The model under review builds one solid part; all positions refer to its coordinate system, in mm. A direction names the side the tool comes from. Round coordinates to 2 decimals unless told otherwise and drop trailing zeros. Return JSON: item names as keys, results as strings. Group by question number.
```python
from build123d import *

# Parameters (mm, degrees)
SKETCH1_R               = 4.7625
BOSS_EXTRUDE2_DEPTH     = 30.48
FILLET1_R               = 3.175
FILLET3_R               = 1.27
FILLET4_R               = 3.175
FILLET5_R               = 1.27
FILLET6_R               = 1.27
BOSS_EXTRUDE9_START     = -30.48
BOSS_EXTRUDE9_DEPTH     = 30.48
CUT_EXTRUDE6_START      = -30.48
CUT_EXTRUDE6_DEPTH      = 30.48
FILLET9_R               = 6.35
CUT_EXTRUDE7_DEPTH      = 44.536935081
CUT_EXTRUDE7_DEPTH_BACK = 44.536935081
BOSS_EXTRUDE11_START    = -30.48
SKETCH4_R               = 4.7625
BOSS_EXTRUDE11_DEPTH    = 30.48
FILLET10_R              = 12.7
FILLET11_R              = 12.7


with BuildPart() as part:
    # Sketch1 → Boss-Extrude2 (new body)
    with BuildSketch(Plane(origin=(0, 0, 0), x_dir=(1, 0, 0), z_dir=(0, 1, 0))):
        with BuildLine():
            Line((11.860213807, -12.884548704), (13.754545104, -18.945407466))
            Line((13.754545104, -18.945407466), (7.404545104, -18.945407466))
            Line((7.404545104, -18.945407466), (6.640447212, -16.500698134))
            ThreePointArc((6.640447212, -16.500698134), (5.961240353, -16.792309403), (5.2705, -17.055438375))
            ThreePointArc((5.2705, -17.055438375), (0, -22.325938375), (-5.2705, -17.055438375))
            ThreePointArc((-5.2705, -17.055438375), (-5.919586773, -14.929400926), (-6.188032569, -12.722755117))
            ThreePointArc((-6.188032569, -12.722755117), (-14.1478, 0), (-6.188032569, 12.722755117))
            ThreePointArc((-6.188032569, 12.722755117), (-5.919586773, 14.929400926), (-5.2705, 17.055438375))
            ThreePointArc((-5.2705, 17.055438375), (0, 22.325938375), (5.2705, 17.055438375))
            ThreePointArc((5.2705, 17.055438375), (12.040379738, 12.314885712), (16.362502035, 5.2705))
            ThreePointArc((16.362502035, 5.2705), (21.633002035, 0), (16.362502035, -5.2705))
            ThreePointArc((16.362502035, -5.2705), (14.592418813, -9.361982053), (11.860213807, -12.884548704))
        make_face()
        with Locations(Location((0, 17.055438375, 0), (0, 0, 90))):
            Circle(SKETCH1_R, mode=Mode.SUBTRACT)
        with Locations(Location((16.362502035, 0, 0), (0, 0, 90))):
            Circle(SKETCH1_R, mode=Mode.SUBTRACT)
        with Locations(Location((0, -17.055438375, 0), (0, 0, 90))):
            Circle(SKETCH1_R, mode=Mode.SUBTRACT)
        with BuildLine():
            Line((5.737156066, -9.353468881), (8.338191551, -17.675407466))
            Line((8.338191551, -17.675407466), (12.027017511, -17.675407466))
            Line((12.027017511, -17.675407466), (8.623309815, -6.785342119))
            ThreePointArc((8.623309815, -6.785342119), (-7.294145861, 8.197424961), (5.737156066, -9.353468881))
        make_face(mode=Mode.SUBTRACT)
    extrude(amount=BOSS_EXTRUDE2_DEPTH)

    # Fillet1
    # the kernel refuses this fillet: 3.175 mm, written as the material it adds along each edge
    with BuildSketch(Plane(origin=(-6.188032569, 0, -12.722755117), x_dir=(-0.8747186698844794, 0, 0.4846310437389738), z_dir=(0, 1, 0))) as fillet1_piece_1:
        with BuildLine():
            CenterArc((1.675106808, -3.170499128), FILLET1_R, 93.05116293, 49.316383357)
            ThreePointArc((-0.839315123, -1.231863693), (-0.401568779, -0.628256415), (0, 0))
            ThreePointArc((0, 0), (0.753054473, -0.020055884), (1.506108946, 0))
        make_face()
    extrude(amount=30.48)
    with BuildSketch(Plane(origin=(-5.2705, 0, -17.055438375), x_dir=(-0.35770128840140486, 0, 0.9338360607065755), z_dir=(0, 1, 0))) as fillet1_piece_2:
        with BuildLine():
            CenterArc((0.51828136, -3.174477714), FILLET1_R, 91.039263795, 15.495369937)
            ThreePointArc((-0.385307362, -0.130770695), (-0.191391238, -0.069105054), (0, 0))
            ThreePointArc((0, 0), (0.230347271, -0.002089143), (0.460694542, 0))
        make_face()
    extrude(amount=30.48)
    with BuildSketch(Plane(origin=(5.2705, 0, -17.055438375), x_dir=(-0.12720688847868244, 0, -0.9918762057452392), z_dir=(0, 1, 0))) as fillet1_piece_3:
        with BuildLine():
            CenterArc((1.744769682, -3.149206953), FILLET1_R, 97.308218729, 47.663807195)
            ThreePointArc((-0.855148612, -1.326832167), (-0.414685297, -0.671723102), (0, 0))
            ThreePointArc((0, 0), (0.670443906, -0.042816458), (1.340887811, 0))
        make_face()
    extrude(amount=30.48)
    with BuildSketch(Plane(origin=(16.362502035, 0, -5.2705), x_dir=(-0.3771647323765371, 0, -0.9261461896759794), z_dir=(0, 1, 0))) as fillet1_piece_4:
        with BuildLine():
            CenterArc((1.804499427, -3.172306197), FILLET1_R, 92.360366346, 49.97819677)
            ThreePointArc((-0.70894152, -1.232399084), (-0.312723775, -0.640214629), (0, 0))
            ThreePointArc((0, 0), (0.8368693, -0.017240341), (1.673738599, 0))
        make_face()
    extrude(amount=30.48)
    with BuildSketch(Plane(origin=(16.362502035, 0, 5.2705), x_dir=(0.9898341628287173, 0, -0.14222633404954374), z_dir=(0, 1, 0))) as fillet1_piece_5:
        with BuildLine():
            CenterArc((1.950776398, -3.142723467), FILLET1_R, 98.176695151, 51.81827723)
            ThreePointArc((-0.798714948, -1.554982197), (-0.380235314, -0.787313176), (0, 0))
            ThreePointArc((0, 0), (0.749603894, -0.053579045), (1.499207787, 0))
        make_face()
    extrude(amount=30.48)
    with BuildSketch(Plane(origin=(11.860213807, 0, 12.884548704), x_dir=(0.29831988928740816, 0, 0.9544659468286695), z_dir=(0, 1, 0))) as fillet1_piece_6:
        with BuildLine():
            CenterArc((1.816465361, 3.175), FILLET1_R, 213.037149694, 56.962850306)
            ThreePointArc((-0.845191928, 1.444044923), (-0.405599886, 0.731970177), (0, 0))
            Line((0, 0), (1.816465361, 0))
        make_face()
    extrude(amount=30.48)
    with BuildSketch(Plane(origin=(5.2705, 0, 17.055438375), x_dir=(0.9268908474954334, 0, -0.37533099636080863), z_dir=(0, 1, 0))) as fillet1_piece_7:
        with BuildLine():
            CenterArc((1.820147869, -3.156511003), FILLET1_R, 96.186334825, 46.370096176)
            ThreePointArc((-0.700651409, -1.226175281), (-0.30907029, -0.636661485), (0, 0))
            ThreePointArc((0, 0), (0.73900137, -0.015364429), (1.47800274, 0))
        make_face()
    extrude(amount=30.48)
    with BuildSketch(Plane(origin=(-5.2705, 0, 17.055438375), x_dir=(0.038601082712793416, 0, 0.999254700471006), z_dir=(0, 1, 0))) as fillet1_piece_8:
        with BuildLine():
            CenterArc((0.52945245, -3.172633674), FILLET1_R, 92.212228742, 15.495369937)
            ThreePointArc((-0.436253651, -0.148061518), (-0.217455401, -0.076009068), (0, 0))
            ThreePointArc((0, 0), (0.203447006, -0.003928101), (0.406894013, 0))
        make_face()
    extrude(amount=30.48)
    # the kernel refuses this fillet: 3.175 mm, written as the material it takes off along each edge
    with BuildSketch(Plane(origin=(5.737156066, -8.75064331, 9.353468881), x_dir=(0.29831988928740744, 0, 0.9544659468286697), z_dir=(0, 1, 0))) as fillet1_2_piece_1:
        with BuildLine():
            CenterArc((3.500257324, -3.175), FILLET1_R, 90, 88.017608619)
            ThreePointArc((0.327157544, -3.065169276), (0.271751922, -1.521038893), (0, 0))
            Line((0, 0), (3.500257324, 0))
        make_face()
    extrude(amount=47.98128662, mode=Mode.SUBTRACT)

    # Fillet3
    fillet3_edges = [part.edges().sort_by_distance(p)[0] for p in [
        (13.754545104, 15.24, 18.945407466),
        (7.404545104, 15.24, 18.945407466),
    ]]
    fillet(fillet3_edges, radius=FILLET3_R)

    # Fillet4
    # the kernel refuses this fillet: 3.175 mm, written as the material it adds along each edge
    with BuildSketch(Plane(origin=(12.027017511, 0, 17.675407466), x_dir=(-0.29831988928740777, 0, -0.9544659468286695), z_dir=(0, 1, 0))) as fillet4_piece_1:
        with BuildLine():
            CenterArc((4.256556411, 3.175), FILLET4_R, 173.746252409, 96.253747591)
            Line((1.100450152, 3.520858762), (1.037328027, 3.527775938))
            ThreePointArc((1.037328027, 3.527775938), (0.489616488, 1.779372694), (-0.060608588, 0.018943313))
            Line((-0.060608588, 0.018943313), (0, -0.0635))
            Line((0, -0.0635), (4.256556411, -0.0635))
            Line((4.256556411, -0.0635), (4.256556411, 0))
        make_face()
    extrude(amount=30.48)

    # Fillet5
    fillet5_edges = [part.edges().sort_by_distance(p)[0] for p in [
        (8.338191551, 15.24, 17.675407466),
    ]]
    fillet(fillet5_edges, radius=FILLET5_R)

    # Fillet6
    fillet6_edges = [part.edges().sort_by_distance(p)[0] for p in [
        (6.640447212, 15.24, 16.500698134),
        (8.623309815, 15.24, 6.785342119),
    ]]
    fillet(fillet6_edges, radius=FILLET6_R)

    # Sketch2 → Boss-Extrude9 (add)
    with BuildSketch(Plane(origin=(0, 30.48, 0), x_dir=(1, 0, 0), z_dir=(0, 1, 0)).offset(BOSS_EXTRUDE9_START)):
        with BuildLine():
            ThreePointArc((7.943426233, 15.662766674), (13.175324303, 14.973004025), (15.611766116, 10.291948459))
            ThreePointArc((15.611766116, 10.291948459), (15.492196473, 9.129027942), (15.138490831, 8.014768839))
            ThreePointArc((15.138490831, 8.014768839), (15.444654673, 7.422560084), (15.731226864, 6.820626626))
            ThreePointArc((15.731226864, 6.820626626), (15.781158654, 6.716236617), (15.834861283, 6.61373547))
            ThreePointArc((15.834861283, 6.61373547), (16.614943687, 8.379799111), (16.881766116, 10.291948459))
            ThreePointArc((16.881766116, 10.291948459), (13.476256049, 16.290071233), (6.580412696, 16.439470316))
            ThreePointArc((6.580412696, 16.439470316), (6.637545403, 16.407150651), (6.69533405, 16.376019005))
            ThreePointArc((6.69533405, 16.376019005), (7.325689413, 16.030433186), (7.943426233, 15.662766674))
        make_face()
    extrude(amount=BOSS_EXTRUDE9_DEPTH)

    # Sketch2<12> → Cut-Extrude6 (cut)
    with BuildSketch(Plane(origin=(0, 30.48, 0), x_dir=(1, 0, 0), z_dir=(0, 1, 0)).offset(CUT_EXTRUDE6_START)):
        with BuildLine():
            ThreePointArc((15.138490831, 8.014768839), (12.043511127, 12.311557951), (7.943426233, 15.662766674))
            ThreePointArc((7.943426233, 15.662766674), (5.173639716, 13.509603196), (4.183683511, 10.143920944))
            ThreePointArc((4.183683511, 10.143920944), (7.605607592, 7.90930294), (9.972426866, 4.577449316))
            ThreePointArc((9.972426866, 4.577449316), (13.062589614, 5.533925069), (15.138490831, 8.014768839))
        make_face()
    extrude(amount=CUT_EXTRUDE6_DEPTH, mode=Mode.SUBTRACT)

    # Fillet9
    fillet9_edges = [part.edges().sort_by_distance(p)[0] for p in [
        (6.580412696, 15.24, -16.439470316),
        (15.834861283, 15.24, -6.61373547),
        (9.972426866, 15.24, -4.577449316),
        (4.183683511, 15.24, -10.143920944),
    ]]
    fillet(fillet9_edges, radius=FILLET9_R)

    # Sketch3 → Cut-Extrude7 (cut, two sides: drawn at the far end of the back side and taken through both)
    with BuildSketch(Plane(origin=(0, 30.48, 0), x_dir=(1, 0, 0), z_dir=(0, 1, 0)).offset(-CUT_EXTRUDE7_DEPTH_BACK)):
        with BuildLine():
            Line((-7.505454184, 11.992847966), (-2.296148987, 12.883016287))
            ThreePointArc((-2.296148987, 12.883016287), (2.423426985, 12.955632538), (4.7625, 17.055438375))
            Line((4.7625, 17.055438375), (9.734184624, 17.275056095))
            ThreePointArc((9.734184624, 17.275056095), (-1.208436668, 22.214922829), (-7.505454184, 11.992847966))
        make_face()
    extrude(amount=CUT_EXTRUDE7_DEPTH + CUT_EXTRUDE7_DEPTH_BACK, mode=Mode.SUBTRACT)

    # Sketch4 → Boss-Extrude11 (add)
    with BuildSketch(Plane(origin=(0, 30.48, 0), x_dir=(1, 0, 0), z_dir=(0, 1, 0)).offset(BOSS_EXTRUDE11_START)):
        with BuildLine():
            ThreePointArc((16.86594215, 9.822043775), (17.712963238, 13.767422556), (19.105519309, 17.554802394))
            ThreePointArc((19.105519309, 17.554802394), (17.767180424, 27.639662161), (9.18901652, 22.17059903))
            ThreePointArc((9.18901652, 22.17059903), (9.198998035, 21.978650402), (9.201259866, 21.786455734))
            ThreePointArc((9.201259866, 21.786455734), (7.906472539, 18.553470941), (4.7625, 17.055438375))
            Line((4.7625, 17.055438375), (9.734184624, 17.275056095))
            ThreePointArc((9.734184624, 17.275056095), (14.943475982, 15.121124841), (16.86594215, 9.822043775))
        make_face()
        with Locations(Location((15.22151652, 22.17059903, 0), (0, 0, 270))):
            Circle(SKETCH4_R, mode=Mode.SUBTRACT)
    extrude(amount=BOSS_EXTRUDE11_DEPTH)

    # Fillet10
    fillet10_edges = [part.edges().sort_by_distance(p)[0] for p in [
        (4.7625, 15.24, -17.055438375),
        (19.105519309, 15.24, -17.554802394),
        (-7.505454184, 15.24, -11.992847966),
    ]]
    fillet(fillet10_edges, radius=FILLET10_R)

    # Fillet11
    # the kernel refuses this fillet: 12.7 mm, written as the material it takes off along each edge
    with BuildSketch(Plane(origin=(-2.296148987, -3.519120011, -12.883016287), x_dir=(0.9377307104980771, 0, 0.3473630875449655), z_dir=(0, 1, 0))) as fillet11_piece_1:
        with BuildLine():
            CenterArc((3.28451201, -12.560548615), FILLET11_R, 98.498560753, 11.829576247)
            Line((-1.127419619, -0.651524335), (-1.215658252, -0.413343849))
            ThreePointArc((-1.215658252, -0.413343849), (-0.690798794, -0.105843114), (-0.127088985, 0.219919053))
            Line((-0.127088985, 0.219919053), (0.03753728, 0.251210972))
            ThreePointArc((0.03753728, 0.251210972), (0.703824002, 0.201705731), (1.370110724, 0.251210972))
            Line((1.370110724, 0.251210972), (1.407648004, 0))
        make_face()
    extrude(amount=37.518240022, mode=Mode.SUBTRACT)


solid = part.part
```
1. Draft analysis for pull direction X (two halves, no side actions). For faces 1 (the face through (12.32, 15.03, 13.04)), 2 (the face through (-10.8, 15.45, -8.73)), 3 (the face through (10.3, 0, 4.4)), 4 (the face through (-0.209, 15.027, 21.813)), state which applies: pulls with the +X half, pulls with the -X half, needs draft (parallel to the pull), parting line crosses it, or undercut.
2. For P1, Ø4, axis at x = 9.5, y = 16, coming from the +Z side; P2, Ø10, axis at x = -3, y = 21.5, coming from the -Z side; P3, Ø5, axis at x = 11, y = 18.5, coming from the -Z side, all flat-tipped, find the tip position at first contact; note any pin that passes through.
3. We need section A-A, the plane y = 5.5. Give the number of separate pieces and of enclosed holes in the cut face, then the cut area to 3 significant figures.
4. Tool access review of faces 5 (the face through (10.813, 15.027, 15.304)), 6 (the face through (7.73, 15.45, 18.79)), 7 (the face through (10.3, 30.48, 4.4)), 8 (the face through (12.815, 15.027, 15.939)): name each direction out of +Z, -Z, +X, -X, +Y, -Y from which nothing blocks a thin tool from reaching the whole face with its end or side.
5. Wall thickness on line 1 (X direction, y = 21, z = 0) (3 decimals); line 2 (Z direction, x = 20.5, y = 2); line 3 (Z direction, x = 15, y = 9): over which ranges is each line inside the solid? List them lowest first.
Check sheet entries:
{
 "1": {"face 1": "pulls with the +X half", "face 2": "pulls with the -X half", "face 3": "needs draft", "face 4": "undercut"},
 "2": {"P1": "stops at z = 18.95", "P2": "stops at z = -12.73", "P3": "stops at z = -27.95"},
 "3": {"separate pieces": "1", "enclosed holes": "4", "area": "345 mm²"},
 "4": {"face 5": "+Y, -Y", "face 6": "+Z, +Y, -Y", "face 7": "+Z, -Z, +X, -X, +Y", "face 8": "+X, +Y, -Y"},
 "5": {"line 1": "x = -14.148 to -10.973, 10.973 to 11.6, 21.125 to 21.633", "line 2": "z = -25.09 to -19.25, -3.26 to -2.36, 2.36 to 3.26", "line 3": "z = -28.2 to -26.93, -17.41 to -12.86, -7.72 to -4.56, 4.56 to 8.63"}
}
